```python
from build123d import *

# Parameters (mm, degrees)
BOSS_EXTRUDE1_DEPTH = 75


with BuildPart() as part:
    # Sketch1 → Boss-Extrude1 (new, symmetric)
    with BuildSketch(Plane(origin=(0, 0, 0), x_dir=(0, 0, -1), z_dir=(1, 0, 0))):
        Polygon((0, 0), (0, -8), (1, -8), (1, -1.5), (8, -1.5), (8, 0), align=None)
    extrude(amount=BOSS_EXTRUDE1_DEPTH, both=True)

    # Mirror2: part across plane


with BuildPart() as part_1:
    add(part.part)
    add(part.part.mirror(Plane(origin=(75, 0, 0), x_dir=(1, 0, 0), z_dir=(0, 0, -1))))


solid = part_1.part
```
The listing builds one solid part. Answer for the finished solid, in the listing's coordinates (mm). A direction names the side the tool comes from. Give positions to 0.01 mm unless a question says otherwise; leave off trailing zeros. Order: outer loops, then holes, each group sorted by start corner. A loop starts at its lowest first (then second) coordinate and runs counter-clockwise, first axis right, second up.
Item 1: The part is cut by section B-B, the plane y = -5.25. Give the vertices of the cut face in (x, z).
From the geometry:
outline: (-75, -1) - (75, -1) - (75, 1) - (-75, 1) - close
Item 2: Which of the six approach directions +Z, -Z, +X, -X, +Y, -Y give full straight-line access (tool end or side, diameter ignored) to faces 1 (the face through (1, -1.5, 4)), 2 (the face through (1, -5, -1)), 3 (the face through (1, 0, 0))?
From the geometry:
face 1: +Z, +X, -X, -Y
face 2: -Z, +X, -X, -Y
face 3: +Z, -Z, +X, -X, +Y
Item 3: Find the intervals of material crossed by probe 1 along Z at (x, y) = (50.5, -5.5); probe 2 along Y at (x, z) = (1, -3), in increasing order.
From the geometry:
probe 1: z = -1 to 1
probe 2: y = -1.5 to 0
Item 4: Given pin 1 Ø2 at (x, z) = (-1.5, 5.5) entering from -Y; pin 2 Ø3 at (x, y) = (-23.5, -5.5) entering from +Z, each flat-ended and moving along its own axis, determine where each tip first touches the part or whether it passes through.
From the geometry:
pin 1: stops at y = -1.5
pin 2: stops at z = 1
Item 5: The part is cut by section A-A, the plane x = 23.5. Give the vertices of the cut face in (y, z).
From the geometry:
outline: (-8, -1) - (-1.5, -1) - (-1.5, -8) - (0, -8) - (0, 8) - (-1.5, 8) - (-1.5, 1) - (-8, 1) - close
Item 6: The part is cut by section C-C, the plane z = 2.5. Give the vertices of the cut face in (x, y), and give its area (3 significant figures).
From the geometry:
outline: (-75, -1.5) - (75, -1.5) - (75, 0) - (-75, 0) - close
area: 225 mm2
